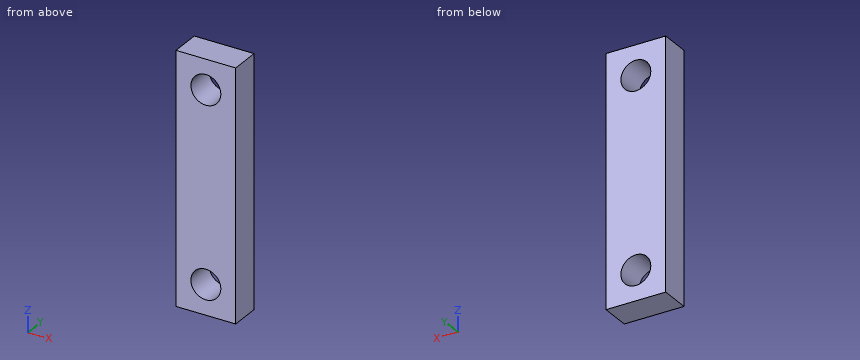
Autodesk Inventor part; units mm, degrees
ref_plane "YZ Plane" through (0, 0, 0) normal (1, 0, 0) x (0, 1, 0)
ref_plane "XZ Plane" through (0, 0, 0) normal (0, 1, 0) x (-1, 0, 0)
ref_plane "XY Plane" through (0, 0, 0) normal (0, 0, 1) x (1, 0, 0)
sketch "Sketch1" plane through (0, 0, 0) normal (0, 1, 0) x (-1, 0, 0)
  line L0 (3, 12.5) -> (-3, 12.5)
  line L1 (-3, 12.5) -> (-3, -12.5)
  line L2 (-3, -12.5) -> (3, -12.5)
  line L3 (3, -12.5) -> (3, 12.5)
  line L4 (3, 12.5) -> (-3, -12.5) construction
  line L5 (-3, 12.5) -> (3, -12.5) construction
  line L6 (-3, -12.5) -> (-3, -9.5)
  line L7 (-3, -9.5) -> (0, -9.5)
  circle A0 centre (0, -9.5) radius 1.5
  line L8 (-3, 12.5) -> (-3, 9.5)
  line L9 (-3, 9.5) -> (0, 9.5)
  circle A1 centre (0, 9.5) radius 1.5
  point P0 (0, 0)
  dimension "d0" = 6
  dimension "d1" = 25
  dimension "d4" = 3
  dimension "d5" = 3
  dimension "d6" = 3
  dimension "d7" = 3
  dimension "d8" = 3
  dimension "d9" = 3
extrude "Extrusion1" add sketch "Sketch1" along normal blind 3 contours A1 | A0 | L3 L2 L1 L0
extrude "Extrusion2" cut sketch "Sketch1" along normal blind 3 contours A0
extrude "Extrusion3" cut sketch "Sketch1" along normal blind 3 contours A1
properties part number "Akrilik Kabel SD Serayu"
Could you check a few things on this model? Use its own coordinates, in mm. Coordinates: 2 decimals unless noted, no trailing zeros. Write each loop counter-clockwise with the first axis right and the second up, starting at its lowest first coordinate (ties: lowest second). Pieces come first, ordered by that corner, then holes. Notation, with made-up numbers: M 11,38 L 53,38 A34 cw 53,77 Z; hole C -7,-16 d4. An arc over 180 degrees is marked long. Answer as CSV lines item,"result". Start each with the question number.
1) I want a section at A-A, the plane z = -9.5. Please give me the cut outline in (x, y).
2) Please list where these lines run through material, in increasing order: line 1 (Z direction, x = 0, y = 0.7); line 2 (X direction, y = 2.2, z = -9.5); line 3 (Z direction, x = 1.1, y = 0.65). Write a range as from..to.
3) I want a section at C-C, the plane x = 0. Please give me the cut outline in (y, z), and give its area (3 significant figures).
4) I want a section at B-B, the plane y = 1.2. Please give me the cut outline in (x, z), and give its area (3 significant figures).
5) For P1, Ø1.8, axis at x = 0, z = 9.5, coming from the -Y side; P2, Ø1, axis at x = 1.5, z = 1.5, coming from the -Y side, each with a flat end and sliding along its axis, tell me the tip position at first contact or that it passes through.
6) I want a section at D-D, the plane x = 1.1. Please give me the cut outline in (y, z).
Data:
1,outline,"M -3,0 L -1.5,0 L -1.5,3 L -3,3 Z; M 1.5,0 L 3,0 L 3,3 L 1.5,3 Z"
2,line 1,"z = -12.5..-11, -8..8, 11..12.5"
2,line 2,"x = -3..-1.5, 1.5..3"
2,line 3,"z = -12.5..-10.52, -8.48..8.48, 10.52..12.5"
3,outline,"M 0,-12.5 L 3,-12.5 L 3,-11 L 0,-11 Z; M 0,-8 L 3,-8 L 3,8 L 0,8 Z; M 0,11 L 3,11 L 3,12.5 L 0,12.5 Z"
3,area,"57.0 mm^2"
4,outline,"M -3,-12.5 L 3,-12.5 L 3,12.5 L -3,12.5 Z; hole C 0,-9.5 d3; hole C 0,9.5 d3"
4,area,"136 mm^2"
5,P1,"passes through"
5,P2,"stops at y = 0"
6,outline,"M 0,-12.5 L 3,-12.5 L 3,-10.52 L 0,-10.52 Z; M 0,-8.48 L 3,-8.48 L 3,8.48 L 0,8.48 Z; M 0,10.52 L 3,10.52 L 3,12.5 L 0,12.5 Z"
